Autodesk Inventor part; units mm, degrees
ref_plane "Work Plane1" through (0, 49.8, 0) normal (0, 1, 0) x (1, 0, 0)
ref_plane "Work Plane2" through (0, 49.8, 0) normal (0, 1, 0) x (1, 0, 0)
ref_plane "Work Plane3" through (0, 20.75, 0) normal (0, -1, 0) x (1, 0, 0)
sketch "Sketch1" plane through (0, 0, 0) normal (1, 0, 0) x (0, 1, 0)
  point P0 (0, 0)
sketch "Sketch2" plane through (0, 0, 0) normal (0, 1, 0) x (-1, 0, 0)
  circle A0 centre (0, 0) radius 2
  dimension "d0" = 4
extrude "Extrusion1" add sketch "Sketch2" along normal blind 25.2
sketch "Sketch3" plane through (0, 25.2, 0) normal (0, 1, 0) x (1, 0, 0)
  circle A0 centre (0, 0) radius 2
  circle A1 centre (0, 0) radius 4.5
  dimension "d3" = 9
extrude "Extrusion2" add sketch "Sketch3" along normal blind 2 contours A0 | A1
sketch "Sketch4" plane through (0, 27.2, 0) normal (0, 1, 0) x (1, 0, 0)
  circle A0 centre (0, 0) radius 4.5
extrude "Extrusion3" add sketch "Sketch4" along normal blind 8.5
sketch "Sketch5" plane through (0, 35.7, 0) normal (0, 1, 0) x (1, 0, 0)
  point P0 (0, 0)
ref_plane "Work Plane1" through (0, 49.8, 0) normal (0, 1, 0) x (1, 0, 0)
sketch "Sketch6" plane through (0, 49.8, 0) normal (0, 1, 0) x (1, 0, 0)
  arc A0 (2.3688, -2.3688) -> (0, -3.35) centre (3.0339, -7.3244) ccw
  arc A1 (0, -3.35) -> (-2.3688, -2.3688) centre (-3.0339, -7.3244) ccw
  arc A2 (3.35, 0) -> (2.3688, -2.3688) centre (7.3244, -3.0339) ccw
  arc A3 (2.3688, 2.3688) -> (3.35, 0) centre (7.3244, 3.0339) ccw
  arc A4 (-3.35, 0) -> (-2.3688, 2.3688) centre (-7.3244, 3.0339) ccw
  arc A5 (-2.3688, -2.3688) -> (-3.35, 0) centre (-7.3244, -3.0339) ccw
  arc A6 (-2.3688, 2.3688) -> (0, 3.35) centre (-3.0339, 7.3244) ccw
  arc A7 (0, 3.35) -> (2.3688, 2.3688) centre (3.0339, 7.3244) ccw
  point P0 (0, 0)
  dimension "d25" = 5
sketch "Sketch7" plane through (0, 35.7, 0) normal (0, 1, 0) x (1, 0, 0)
  circle A0 centre (0, 0) radius 4.5
  circle A1 centre (0, 0) radius 4.5
  arc A2 (-3.1879, -3.176) -> (-4.5, 0.0084) centre (-8.1841, -3.372) ccw
  arc A3 (-4.5, 0.0084) -> (-3.176, 3.1879) centre (-8.1714, 3.4027) ccw
  arc A4 (4.5, -0.0084) -> (3.176, -3.1879) centre (8.1714, -3.4027) ccw
  arc A5 (3.1879, 3.176) -> (4.5, -0.0084) centre (8.1841, 3.372) ccw
  arc A6 (-0.0084, -4.5) -> (-3.1879, -3.176) centre (-3.4027, -8.1714) ccw
  arc A7 (3.176, -3.1879) -> (-0.0084, -4.5) centre (3.372, -8.1841) ccw
  arc A8 (0.0084, 4.5) -> (3.1879, 3.176) centre (3.4027, 8.1714) ccw
  arc A9 (-3.176, 3.1879) -> (0.0084, 4.5) centre (-3.372, 8.1841) ccw
  circle A10 centre (0, 0) radius 4.5
extrude "Extrusion4" cut sketch "Sketch7" against normal blind 8.5 contours A0 A5 | A8 A0 | A0 A4 | A9 A0 | A0 A7 | A3 A0 | A0 A6 | A2 A0
ref_plane "Work Plane2" through (0, 49.8, 0) normal (0, 1, 0) x (1, 0, 0)
loft "Loft2" add profiles "Sketch6" section 2 edges at (-1.4806, 35.7, 3.5556) (1.4672, 35.7, 3.5611) (3.5556, 35.7, 1.4806) (3.5611, 35.7, -1.4672) (1.4806, 35.7, -3.5556) (-1.4672, 35.7, -3.5611) (-3.5556, 35.7, -1.4806) (-3.5611, 35.7, 1.4672)
sketch "Sketch10" plane through (0, 27.2, 0) normal (0, 1, 0) x (1, 0, 0)
  arc A0 (3.176, -3.1879) -> (-0.0084, -4.5) centre (3.372, -8.1841) ccw
  arc A1 (-0.0084, -4.5) -> (3.176, -3.1879) centre (0, 0) ccw
  arc A2 (-0.0084, -4.5) -> (-3.1879, -3.176) centre (-3.4027, -8.1714) ccw
  arc A3 (-0.0084, -4.5) -> (-3.1879, -3.176) centre (-3.4027, -8.1714) ccw
  arc A4 (-3.1879, -3.176) -> (-0.0084, -4.5) centre (0, 0) ccw
  arc A5 (-3.1879, -3.176) -> (-4.5, 0.0084) centre (-8.1841, -3.372) ccw
  arc A6 (-4.5, 0.0084) -> (-3.1879, -3.176) centre (0, 0) ccw
  arc A7 (-4.5, 0.0084) -> (-3.176, 3.1879) centre (-8.1714, 3.4027) ccw
  arc A8 (-3.176, 3.1879) -> (-4.5, 0.0084) centre (0, 0) ccw
  arc A9 (-3.176, 3.1879) -> (0.0084, 4.5) centre (-3.372, 8.1841) ccw
  arc A10 (-3.176, 3.1879) -> (0.0084, 4.5) centre (-3.372, 8.1841) ccw
  arc A11 (0.0084, 4.5) -> (-3.176, 3.1879) centre (0, 0) ccw
  arc A12 (0.0084, 4.5) -> (3.1879, 3.176) centre (3.4027, 8.1714) ccw
  arc A13 (3.1879, 3.176) -> (0.0084, 4.5) centre (0, 0) ccw
  arc A14 (3.1879, 3.176) -> (4.5, -0.0084) centre (8.1841, 3.372) ccw
  arc A15 (4.5, -0.0084) -> (3.1879, 3.176) centre (0, 0) ccw
  arc A16 (4.5, -0.0084) -> (3.176, -3.1879) centre (8.1714, -3.4027) ccw
  arc A17 (3.176, -3.1879) -> (4.5, -0.0084) centre (0, 0) ccw
extrude "Extrusion5" cut sketch "Sketch10" against normal blind 10 contours A1 A0 | A16 A17 | A4 A2 | A14 A15 | A6 A5 | A12 A13 | A8 A7 | A9 A11
sketch "Sketch11" plane through (0, 25.2, 0) normal (0, -1, 0) x (1, 0, 0)
  point P0 (0, 0)
ref_plane "Work Plane3" through (0, 20.75, 0) normal (0, -1, 0) x (1, 0, 0)
sketch "Sketch12" plane through (0, 20.75, 0) normal (0, -1, 0) x (1, 0, 0)
  circle A0 centre (0, 0) radius 2
  circle A1 centre (0, 0) radius 3.5
  dimension "d33" = 7
extrude "Extrusion6" add sketch "Sketch12" against normal blind 1
fillet "Fillet1" radius 0.5 1 edges at (-3.5, 21.75, 0)
sketch "Sketch13" plane through (0, 20.75, 0) normal (0, -1, 0) x (1, 0, 0)
  arc A0 (3.176, 3.1879) -> (4.5, 0.0084) centre (8.1714, 3.4027) ccw
  arc A1 (-0.0084, 4.5) -> (3.176, 3.1879) centre (3.372, 8.1841) ccw
  arc A2 (-3.1879, 3.176) -> (-0.0084, 4.5) centre (-3.4027, 8.1714) ccw
  arc A3 (-4.5, -0.0084) -> (-3.1879, 3.176) centre (-8.1841, 3.372) ccw
  arc A4 (-3.176, -3.1879) -> (-4.5, -0.0084) centre (-8.1714, -3.4027) ccw
  arc A5 (0.0084, -4.5) -> (-3.176, -3.1879) centre (-3.372, -8.1841) ccw
  arc A6 (3.1879, -3.176) -> (0.0084, -4.5) centre (3.4027, -8.1714) ccw
  arc A7 (4.5, 0.0084) -> (3.1879, -3.176) centre (8.1841, -3.372) ccw
  circle A8 centre (0, 0) radius 2
extrude "Extrusion7" add sketch "Sketch13" against normal blind 10
ref_plane "Work Plane4" through (3.0339, 53.55, 7.3244) normal (0, 1, 0) x (0.9238795, 0, -0.3826834)
sketch "Sketch16" plane through (3.0339, 53.55, 7.3244) normal (0, 1, 0) x (0.9238795, 0, -0.3826834)
  arc A0 (1.282, 4.8329) -> (-1.282, 4.8329) centre (0, 0) ccw
  arc A1 (3.095, 6.6459) -> (1.282, 4.8329) centre (5.6058, 2.322) ccw
  arc A2 (3.095, 9.2098) -> (3.095, 6.6459) centre (7.9279, 7.9279) ccw
  arc A3 (1.282, 11.0228) -> (3.095, 9.2098) centre (5.6058, 13.5337) ccw
  arc A4 (-1.282, 11.0228) -> (1.282, 11.0228) centre (0, 15.8557) ccw
  arc A5 (-3.095, 9.2098) -> (-1.282, 11.0228) centre (-5.6058, 13.5337) ccw
  arc A6 (-3.095, 6.6459) -> (-3.095, 9.2098) centre (-7.9279, 7.9279) ccw
  arc A7 (-1.282, 4.8329) -> (-3.095, 6.6459) centre (-5.6058, 2.322) ccw
  point P0 (0, 7.9279)
  point P1 (0, 7.9279)
loft "Loft4" add section 1 edges at (1.1204, 49.8, 2.705) (2.705, 49.8, 1.1204) (2.705, 49.8, -1.1204) (1.1204, 49.8, -2.705) (-1.1204, 49.8, -2.705) (-2.705, 49.8, -1.1204) (-2.705, 49.8, 1.1204) (-1.1204, 49.8, 2.705) section 2 point at (0, 53.55, 0)
properties part number "mixer" material "PBT Plastic"
Geometry: final body of the model. Coordinates: model frame, mm. A direction names the side the tool comes from. Coordinates: 2 decimals unless noted, no trailing zeros. Loops run counter-clockwise (first coordinate to the right, second up) from the corner with the lowest first, then second, coordinate; pieces in that order, holes last. Notation, with made-up numbers: (-33, 11.25) - (3, 11.25) arc R8 ccw to (3, 20.25) - close; hole circle Ø3 at (65.25, 54). An arc over 180 degrees is marked (long way). Put each result on its own line as item: value. Start each with the question number.
Q1. Cut plane A-A, the plane y = 30.5. Return loops of the section in (x, z), and give its area (3 significant figures).
Q2. Cut plane B-B, the plane y = 13. Return loops of the section in (x, z), and give its area (3 significant figures).
Q3. Set-up query: faces 1 (the flat face through (-2, 20.75, 1)), 2 (the cylindrical face through (1.445, 22.944, 3.571)). Return all of +Z, -Z, +X, -X, +Y, -Y with unobstructed straight access to the full face (end or side cutting, diameter ignored); none if empty.
Q4. Pin query (flat end, axial travel): pin 1 Ø1.5 at (x, z) = (-0.5, -2.5) entering from +Y; pin 2 Ø1.5 at (x, y) = (2, 14.5) entering from +Z; pin 3 Ø4 at (y, z) = (18, 2.5) entering from -X. Return the tip coordinate at first contact, or that it passes through.
Q5. Line query: line 1 (X direction, y = 28.5, z = 3); line 2 (Z direction, x = -3, y = 36); line 3 (Y direction, x = 0.5, z = 0.75). Output: solid intervals per line, ascending.
Filled sheet:
1. outline: (-4.5, -0.01) arc R5 cw to (-3.18, -3.19) arc R5 cw to (0.01, -4.5) arc R5 cw to (3.19, -3.18) arc R5 cw to (4.5, 0.01) arc R5 cw to (3.18, 3.19) arc R5 cw to (-0.01, 4.5) arc R5 cw to (-3.19, 3.18) arc R5 cw to start
1. area: 51.6 mm²
2. outline: circle Ø4 at (0, 0)
2. area: 12.6 mm²
3. face 1: -Y
3. face 2: +Z, +X, +Y, -Y
4. pin 1: y = 51.38
4. pin 2: z = 1.56
4. pin 3: x = -1.94
5. line 1: -3.2 to 3.19
5. line 2: -3.18 to 3.17
5. line 3: 0 to 52.43
